```python
from build123d import *

# Parameters (mm, degrees)
EXTRUDE_1_DEPTH          = 5
SKETCH_3_W               = 5
SKETCH_3_H               = 50
CUT_EXTRUDE_1_DEPTH      = 692.252839152
CUT_EXTRUDE_1_DEPTH_BACK = 692.252839152
SKETCH_5_R               = 2
SKETCH_7_R               = 6
CUT_EXTRUDE_2_DEPTH      = 692.25283929
SKETCH_2_W               = 20
SKETCH_2_H               = 5
SKETCH_8_R               = 6
CUT_EXTRUDE_3_DEPTH      = 346.118964709
CUT_EXTRUDE_4_DEPTH      = 346.897812083
CUT_EXTRUDE_4_DEPTH_BACK = 346.897812083
SKETCH_9_R               = 2
SCALE_1_SCALE            = 0.5


with BuildPart() as part:
    # 草图1 → 凸台-拉伸1 (new body)
    with BuildSketch(Plane.XY.offset(5)):
        with BuildLine():
            Line((-531.259329651, 335.424320593), (-597.842921786, 202.257136323))
            ThreePointArc((-597.842921786, 202.257136323), (-596.967394134, 182.798242171), (-579.954377966, 173.312864413))
            Line((-579.954377966, 173.312864413), (-512.315057741, 173.312864413))
            Line((-512.315057741, 173.312864413), (-512.315057741, 330.952184638))
            ThreePointArc((-512.315057741, 330.952184638), (-520.017528536, 340.684674533), (-531.259329651, 335.424320593))
        make_face()
    extrude(amount=EXTRUDE_1_DEPTH)

    # 草图3 → 旋转1 (revolve)
    with BuildSketch(Plane(origin=(-559.177191958, 279.588595979, 0), x_dir=(0, 0, 1), z_dir=(-0.894427190999916, 0.4472135954999579, 0))):
        with Locations((7.5, -42.016481195)):
            Rectangle(SKETCH_3_W, SKETCH_3_H)
    revolve(axis=Axis((-566.787193696, 264.368592503, 5), (-0.447213595499958, -0.894427190999916, 0)))

    # 草图5 → 切除-拉伸1 (cut, two sides: drawn at the far end of the back side and taken through both)
    with BuildSketch(Plane(origin=(-7.610001738, -15.220003476, 0), x_dir=(0.894427190999916, -0.4472135954999579, 0), z_dir=(0.4472135954999579, 0.894427190999916, 0)).offset(-CUT_EXTRUDE_1_DEPTH_BACK)):
        with Locations(Location((-625.179106343, -5, 0), (0, 0, 270))):
            Circle(SKETCH_5_R)
    extrude(amount=CUT_EXTRUDE_1_DEPTH + CUT_EXTRUDE_1_DEPTH_BACK, mode=Mode.SUBTRACT)

    # 草图7 → 切除-拉伸2 (cut, through all)
    with BuildSketch(Plane(origin=(-7.610001738, -15.220003476, 0), x_dir=(0.894427190999916, -0.4472135954999579, 0), z_dir=(0.4472135954999579, 0.894427190999916, 0))):
        with Locations((-625.179106343, -5)):
            Circle(SKETCH_7_R)
    extrude(amount=CUT_EXTRUDE_2_DEPTH, mode=Mode.SUBTRACT)

    # 草图2 → 旋转2 (revolve)
    with BuildSketch(Plane.XZ.offset(-173.312864413)):
        with Locations((-558.634717854, 7.5)):
            Rectangle(SKETCH_2_W, SKETCH_2_H)
    revolve(axis=Axis((-548.634717854, 173.312864413, 10), (-1, 0, 0)))

    # 草图8 → 切除-拉伸3 (cut, through all)
    with BuildSketch(Plane(origin=(-548.634717854, 0, 0), x_dir=(0, 0, -1), z_dir=(1, 0, 0))):
        with Locations((-10, 173.312864413)):
            Circle(SKETCH_8_R)
    extrude(amount=CUT_EXTRUDE_3_DEPTH, mode=Mode.SUBTRACT)

    # 草图9 → 切除-拉伸4 (cut, two sides: drawn at the far end of the back side and taken through both)
    with BuildSketch(Plane.ZY.offset(568.634717854).offset(-CUT_EXTRUDE_4_DEPTH_BACK)):
        with Locations((10, 173.312864413)):
            Circle(SKETCH_9_R)
    extrude(amount=CUT_EXTRUDE_4_DEPTH + CUT_EXTRUDE_4_DEPTH_BACK, mode=Mode.SUBTRACT)


with BuildPart() as part_1:
    # 缩放比例1: scaled about (0, 0, 0)
    add(part.part.scale(SCALE_1_SCALE))


solid = part_1.part
```
CAD build for the part. Positions are in the model's coordinates, mm. A direction names the side the tool comes from. Round coordinates to 2 decimals unless told otherwise and drop trailing zeros. Return JSON: item names as keys, results as strings. Group by question number.
(1) Tool access for faces 1 (the flat face through (-287, 86.656, 3)), 2 (the cylindrical face through (-265.36, 89.29, 3.56)), 3 (the flat face through (-284.317, 86.62, 6.15)), 4 (the flat face through (-295.102, 110.088, 1.424)): list every direction of +Z, -Z, +X, -X, +Y, -Y with a clear straight run to the whole face (end or side of a thin tool).
(2) Mould opens along X. For faces 5 (the flat face through (-283.204, 132.09, 3.646)), 6 (the cylindrical face through (-289.56, 117.97, 3.04)), 7 (the flat face through (-296.717, 105.537, 4.24)), 8 (the flat face through (-274.317, 88, 4)) say: +X half, -X half, draft (parallel to the pull), parting line (faces both ways), or undercut.
(3) Wall check: probe 1 along Z at (x, y) = (-275.5, 134); probe 2 along Y at (x, z) = (-267, 3.5); probe 3 along X at (y, z) = (133.5, 3.5). Give the ranges that are in metal, low to high. Write a range as [from, to].
(4) Drop flat-ended pins along their axis: P1, Ø3, axis at x = -275, z = 3, coming from the -Y side; P2, Ø1.2, axis at y = 86.66, z = 5, coming from the -X side; P3, Ø4, axis at y = 87.5, z = 4, coming from the -X side; P4, Ø3, axis at y = 122.5, z = 2.5, coming from the -X side. Give the stop position or say it passes through.
Answer list:
{
 "1": {"face 1": "+Z, -Z, -X, -Y", "face 2": "+Z, +X, -Y", "face 3": "+Z, -X, -Y", "face 4": "-Z, -X"},
 "2": {"face 5": "undercut", "face 6": "undercut", "face 7": "-X half", "face 8": "+X half"},
 "3": {"probe 1": "[2.5, 5]", "probe 2": "[89.25, 158.65]", "probe 3": "[-279.57, -256.16]"},
 "4": {"P1": "y = 84.21", "P2": "through", "P3": "x = -296.96", "P4": "x = -291.78"}
}
